Geometry check sheet. Reference: drawing and pictorial views, mm from the part's lowest x, y, z. Give positions to 0.01 mm unless a question says otherwise; leave off trailing zeros. Write each loop counter-clockwise with the first axis right and the second up, starting at its lowest first coordinate (ties: lowest second). Pieces come first, ordered by that corner, then holes. Notation, with made-up numbers: (81.25, 12.25) -> (94.25, 12.25) arc R33 cw to (94.25, 45.25) -> close; hole circle Ø2 at (29, 85). An arc over 180 degrees is marked (long way). Return JSON: item names as keys, results as strings.
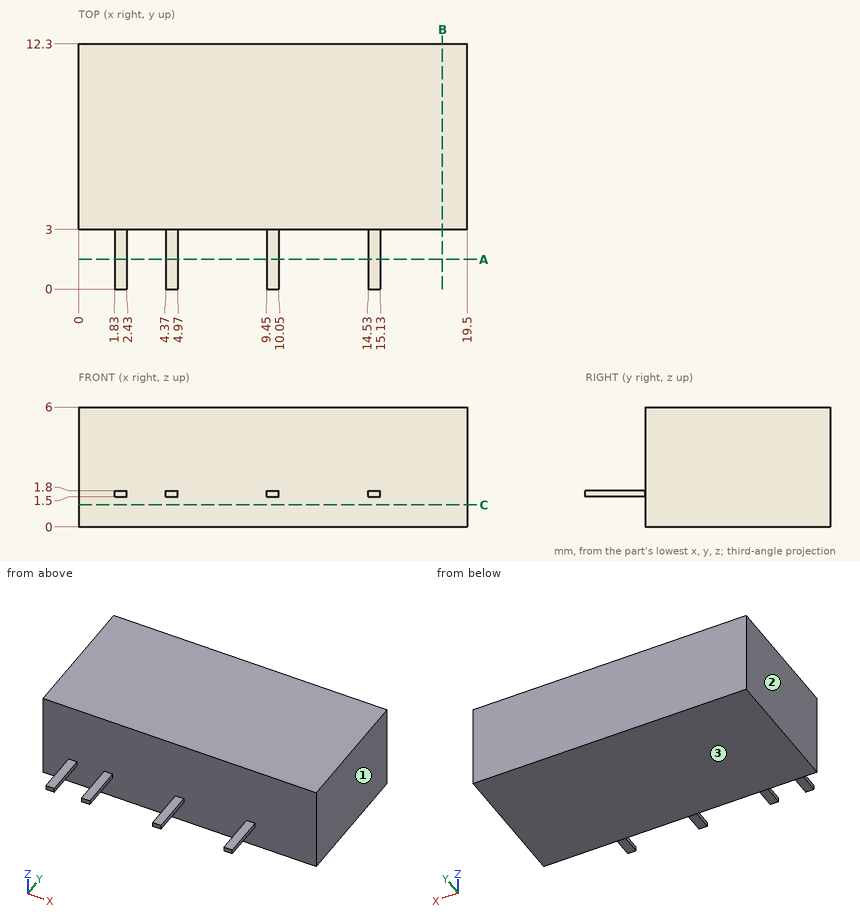
(1) Cross-section at A-A on y = 1.5. Enter the section's corners in (x, z).
Reply:
{"outline": "(1.83, 1.5) -> (2.43, 1.5) -> (2.43, 1.8) -> (1.83, 1.8) -> close; (4.37, 1.5) -> (4.97, 1.5) -> (4.97, 1.8) -> (4.37, 1.8) -> close; (9.45, 1.5) -> (10.05, 1.5) -> (10.05, 1.8) -> (9.45, 1.8) -> close; (14.53, 1.5) -> (15.13, 1.5) -> (15.13, 1.8) -> (14.53, 1.8) -> close"}
(2) Cross-section at C-C on z = 1.1. Enter the section's corners in (x, y).
Reply:
{"outline": "(0, 3) -> (19.5, 3) -> (19.5, 12.3) -> (0, 12.3) -> close"}
(3) Depth check by flat-ended pin: pin 1 Ø1 at (y, z) = (10, 3) entering from -X; pin 2 Ø0.5 at (x, y) = (2, 1) entering from -Z; pin 3 Ø0.7 at (x, y) = (4.5, 1.5) entering from +Z. Enter the tip coordinate at first touch or a pass-through.
Reply:
{"pin 1": "x = 0", "pin 2": "z = 1.5", "pin 3": "z = 1.8"}
(4) Release check for a two-part mould opening along X. For the marked faces 1, 2 and 3 record: pulls with the +X half, pulls with the -X half, needs draft (parallel to the pull), parting line crosses it, or undercut.
Reply:
{"face 1": "pulls with the +X half", "face 2": "pulls with the -X half", "face 3": "needs draft"}
(5) Thickness scan on L1, parallel to Y at x = 18.5, z = 2.7. Record the ranges inside material, lowest first.
Reply:
{"L1": "3 to 12.3"}
(6) Cross-section at B-B on x = 18.25. Enter the section's corners in (y, z).
Reply:
{"outline": "(3, 0) -> (12.3, 0) -> (12.3, 6) -> (3, 6) -> close"}
